from build123d import *

# Parameters (mm, degrees)
RESSALTO_EXTRUS_O1_DEPTH = 34
CASCA1_T                 = -2
ESBO_O2_W                = 50
ESBO_O2_H                = 30
CORTE_EXTRUS_O1_DEPTH    = 50
ESBO_O3_R                = 7.5
CORTE_EXTRUS_O2_DEPTH    = 50
ESBO_O6_W                = 36.535898385
ESBO_O6_H                = 30
CORTE_EXTRUS_O5_DEPTH    = 2
ESBO_O7_W                = 21.524791386
ESBO_O7_H                = 30
CORTE_EXTRUS_O6_DEPTH    = 2
CORTE_EXTRUS_O7_DEPTH    = 2


with BuildPart() as part:
    # Esboço1 → Ressalto-extrusão1 (new body)
    with BuildSketch(Plane.XY):
        Polygon((27.679491924, -15), (45, 15), (-45, 15), (-45, -15), align=None)
    extrude(amount=RESSALTO_EXTRUS_O1_DEPTH)

    # Casca1
    casca1_openings = [part.faces().sort_by_distance(p)[0] for p in [
        (-45, 0, 17),
    ]]
    offset(amount=CASCA1_T, openings=casca1_openings, kind=Kind.INTERSECTION)

    # Esboço2 → Corte-extrusão1 (cut)
    with BuildSketch(Plane(origin=(0, 15, 0), x_dir=(1, 0, 0), z_dir=(0, 1, 0))):
        with Locations((-20, -17)):
            Rectangle(ESBO_O2_W, ESBO_O2_H)
    extrude(amount=-CORTE_EXTRUS_O1_DEPTH, mode=Mode.SUBTRACT)

    # Esboço3 → Corte-extrusão2 (cut)
    with BuildSketch(Plane(origin=(0, 0, 0), x_dir=(-1, 0, 0), z_dir=(0, 0, -1))):
        with Locations((20, 0)):
            Circle(ESBO_O3_R)
    extrude(amount=-CORTE_EXTRUS_O2_DEPTH, mode=Mode.SUBTRACT)

    # Esboço6 → Corte-extrusão5 (cut)
    with BuildSketch(Plane(origin=(0, 13, 0), x_dir=(-1, 0, 0), z_dir=(0, -1, 0))):
        with Locations((-23.267949193, -17)):
            Rectangle(ESBO_O6_W, ESBO_O6_H)
    extrude(amount=-CORTE_EXTRUS_O5_DEPTH, mode=Mode.SUBTRACT)

    # Esboço7 → Corte-extrusão6 (cut)
    with BuildSketch(Plane(origin=(0, -13, 0), x_dir=(1, 0, 0), z_dir=(0, 1, 0))):
        with Locations((15.762395693, -17)):
            Rectangle(ESBO_O7_W, ESBO_O7_H)
    extrude(amount=-CORTE_EXTRUS_O6_DEPTH, mode=Mode.SUBTRACT)

    # Esboço8 → Corte-extrusão7 (cut)
    with BuildSketch(Plane(origin=(25.522758664, -14.735571585, 0), x_dir=(0, 0, 1), z_dir=(-0.86602540378444, 0.49999999999999784, 0))):
        with BuildLine():
            ThreePointArc((24.5, 17.015172443), (22.303300859, 22.318473302), (17, 24.515172443))
            Line((17, 24.515172443), (17, 9.515172443))
            ThreePointArc((17, 9.515172443), (22.303300859, 11.711871584), (24.5, 17.015172443))
        make_face()
        with BuildLine():
            Line((17, 9.515172443), (17, 24.515172443))
            ThreePointArc((17, 24.515172443), (9.5, 17.015172443), (17, 9.515172443))
        make_face()
    extrude(amount=-CORTE_EXTRUS_O7_DEPTH, mode=Mode.SUBTRACT)


solid = part.part
CAD build for the part. Positions are in the model's coordinates, mm. A direction names the side the tool comes from. Give positions to 0.01 mm unless a question says otherwise; leave off trailing zeros. Write each loop counter-clockwise with the first axis right and the second up, starting at its lowest first coordinate (ties: lowest second). Pieces come first, ordered by that corner, then holes. Notation, with made-up numbers: (86.25, 5.5) - (134.25, 5.5) arc R16 cw to (134.25, 32.5) - close; hole circle Ø6 at (14, -20). An arc over 180 degrees is marked (long way). Answer as CSV lines item,"result".
Q1. Flat gauge pins, fed straight in: pin 1 Ø2 at (y, z) = (-14, 13.5) entering from -X; pin 2 Ø0.6 at (y, z) = (13.5, 23) entering from -X; pin 3 Ø1 at (y, z) = (1, 8) entering from -X. Where does each tip first touch, or does it go through?
Result set:
pin 1,"x = 26.52"
pin 2,"x = 41.54"
pin 3,"x = 34.32"
Q2. Band-saw the part on D-D (y = 8.5). Give the cut face in (x, z).
Result set:
outline,"(-45, 0) - (41.25, 0) - (41.25, 34) - (-45, 34) - (-45, 32) - (38.94, 32) - (38.94, 2) - (-45, 2) - close"
Q3. Drill centre lines: line 1 (Z direction, x = 24, y = 13.25); line 2 (Y direction, x = -20, z = 1.45); line 3 (X direction, y = -11, z = 21.5). Where is each one in solid material? Low to high. Write a range as from..to.
Result set:
line 1,"0..2, 32..34"
line 2,"-15..-7.5, 7.5..15"
line 3,"27.68..29.99"
Q4. Band-saw the part on A-A (x = 2.5). Give the cut face in (y, z), and give its area (3 significant figures).
Result set:
outline,"(-15, 0) - (15, 0) - (15, 2) - (-15, 2) - close; (-15, 32) - (15, 32) - (15, 34) - (-15, 34) - close"
area,"120 mm²"
Q5. Band-saw the part on B-B (z = 16). Give the cut face in (x, y), and give its area (4 significant figures).
Result set:
outline,"(26.52, -15) - (27.68, -15) - (32.05, -7.44) - (30.31, -6.44) - (26.52, -13) - close; (37.75, 6.44) - (39.48, 5.44) - (45, 15) - (41.54, 15) - (41.54, 13) - close"
area,"39.55 mm²"
Q6. 3-axis set-ups, long thin cutter, end or side, ignore diameter. For faces 4 (the face through (26.525, -14, 17)), 5 (the face through (-12.507, 0.33, 0.986)), 6 (the face through (32.26, -3.07, 10.12)): which of +Z, -Z, +X, -X, +Y, -Y reach the whole face in a straight line?
Result set:
face 4,"-X, +Y, -Y"
face 5,"+Z, -Z"
face 6,"-X, +Y"
Q7. Band-saw the part on C-C (x = -20). Give the cut face in (y, z).
Result set:
outline,"(-15, 0) - (-7.5, 0) - (-7.5, 2) - (-15, 2) - close; (-15, 32) - (-7.5, 32) - (-7.5, 34) - (-15, 34) - close; (7.5, 0) - (15, 0) - (15, 2) - (7.5, 2) - close; (7.5, 32) - (15, 32) - (15, 34) - (7.5, 34) - close"
Q8. Pull direction Z, two halves, no side cores. Call faces 1 (the face through (-2, 0, 32)), 2 (the face through (-1, 0, 0)), 3 (the face through (-45, 0, 1)): released by +Z, released by -Z, zero draft, split by the parting line, or undercut.
Result set:
face 1,"undercut"
face 2,"released by -Z"
face 3,"zero draft"
